```python
from build123d import *

# Parameters (mm, degrees)
SKETCH1_W           = 31.8
SKETCH1_H           = 48
BOSS_EXTRUDE1_DEPTH = 15.8
SKETCH2_R           = 7.62
CUT_EXTRUDE1_DEPTH  = 12.7
SKETCH3_R           = 2.77815
SKETCH3_R_2         = 1.8415
CUT_EXTRUDE2_DEPTH  = 12.7
CUT_EXTRUDE3_DEPTH  = 1.905
SKETCH5_R           = 2.4
BOSS_EXTRUDE2_DEPTH = 1.905
SKETCH6_W           = 29.36
SKETCH6_H           = 13.36
SKETCH6_R           = 3.2605
CUT_EXTRUDE4_DEPTH  = 1.905


with BuildPart() as part:
    # Sketch1 → Boss-Extrude1 (new body)
    with BuildSketch(Plane.XY):
        Rectangle(SKETCH1_W, SKETCH1_H)
    extrude(amount=BOSS_EXTRUDE1_DEPTH)

    # Sketch2 → Cut-Extrude1 (cut)
    with BuildSketch(Plane.XY.offset(15.8)):
        with Locations((0, 8.6)):
            Circle(SKETCH2_R)
        with BuildLine():
            Line((4.7625, -4.1), (4.7625, -16.8))
            ThreePointArc((4.7625, -16.8), (0, -21.5625), (-4.7625, -16.8))
            Line((-4.7625, -16.8), (-4.7625, -4.1))
            ThreePointArc((-4.7625, -4.1), (0, 0.6625), (4.7625, -4.1))
        make_face()
    extrude(amount=-CUT_EXTRUDE1_DEPTH, mode=Mode.SUBTRACT)

    # Sketch3 → Cut-Extrude2 (cut)
    with BuildSketch(Plane(origin=(0, 0, 0), x_dir=(-1, 0, 0), z_dir=(0, 0, -1))):
        with Locations((0, 8.6)):
            Circle(SKETCH3_R)
        with Locations((0, -4.1)):
            Circle(SKETCH3_R_2)
        with Locations((0, -16.8)):
            Circle(SKETCH3_R_2)
    extrude(amount=-CUT_EXTRUDE2_DEPTH, mode=Mode.SUBTRACT)

    # Sketch4 → Cut-Extrude3 (cut)
    with BuildSketch(Plane(origin=(0, 0, 0), x_dir=(-1, 0, 0), z_dir=(0, 0, -1))):
        with BuildLine():
            Line((4.7625, -16.8), (4.7625, -4.1))
            ThreePointArc((4.7625, -4.1), (0, 0.6625), (-4.7625, -4.1))
            Line((-4.7625, -4.1), (-4.7625, -16.8))
            ThreePointArc((-4.7625, -16.8), (0, -21.5625), (4.7625, -16.8))
        make_face()
    extrude(amount=-CUT_EXTRUDE3_DEPTH, mode=Mode.SUBTRACT)

    # Sketch5 → Boss-Extrude2 (add)
    with BuildSketch(Plane.XZ.offset(24)):
        with Locations((-12, 11.9)):
            Circle(SKETCH5_R)
        with Locations((-12, 3.9)):
            Circle(SKETCH5_R)
        with Locations((-4, 11.9)):
            Circle(SKETCH5_R)
        with Locations((-4, 3.9)):
            Circle(SKETCH5_R)
        with Locations((4, 11.9)):
            Circle(SKETCH5_R)
        with Locations((4, 3.9)):
            Circle(SKETCH5_R)
        with Locations((12, 11.9)):
            Circle(SKETCH5_R)
        with Locations((12, 3.9)):
            Circle(SKETCH5_R)
    extrude(amount=BOSS_EXTRUDE2_DEPTH)

    # Sketch6 → Cut-Extrude4 (cut)
    with BuildSketch(Plane(origin=(0, 24, 0), x_dir=(1, 0, 0), z_dir=(0, 1, 0))):
        with Locations((0, -7.9)):
            Rectangle(SKETCH6_W, SKETCH6_H)
        with Locations((-8, -7.9)):
            Circle(SKETCH6_R, mode=Mode.SUBTRACT)
        with Locations((0, -7.9)):
            Circle(SKETCH6_R, mode=Mode.SUBTRACT)
        with Locations((8, -7.9)):
            Circle(SKETCH6_R, mode=Mode.SUBTRACT)
    extrude(amount=-CUT_EXTRUDE4_DEPTH, mode=Mode.SUBTRACT)


solid = part.part
```
Verification items for the finished model (mm, model axes). A direction names the side the tool comes from. Give positions to 0.01 mm unless a question says otherwise; leave off trailing zeros. Order: outer loops, then holes, each group sorted by start corner. A loop starts at its lowest first (then second) coordinate and runs counter-clockwise, first axis right, second up. Notation, with made-up numbers: (30.5, -28.5) - (71.5, -28.5) arc R14 cw to (71.5, -15.5) - close; hole circle Ø10 at (84, -26). An arc over 180 degrees is marked (long way). Answer as CSV lines item,"result". Start each with the question number.
Item 1: Access from +Z, -Z, +X, -X, +Y, -Y to the whole of each face (thin tool, end or side, straight path). Record for faces 1 (the face through (11.48, -24.939, 1.557)), 2 (the face through (-14.68, 23, 8)), 3 (the face through (4.762, -10, 1)).
Item 2: Section check A-A, the plane y = 8.6. Record the boundary of the cut face in (x, z), plus the area to 3 significant figures.
Item 3: Section check B-B, the plane z = 11.9. State how many separate pieces and enclosed holes the cut face has, plus the area to 3 significant figures.
Item 4: Material ranges on L1, parallel to Y at x = 0, z = 7.25; L2, parallel to Y at x = 0, z = 1.45 (1 decimal); L3, parallel to Y at x = 0, z = 2.55 (1 decimal), recorded low to high.
Item 5: Section check C-C, the plane x = -13. Record the boundary of the cut face in (y, z) (3 decimals).
Item 6: Mould release check, pull along Y, two halves, no side actions. Record for faces 4 (the face through (0, -10, 3.1)), 5 (the face through (0, 23, 14.58)), 6 (the face through (0, 24, 8)): released by +Y, released by -Y, zero draft, split by the parting line, or undercut.
Item 7: Gauge pin test, flat ends, axial feed: pin 1 (8 mm diameter, centred on x = -6, z = 12.5, fed in from +Y); pin 2 (7.5 mm diameter, centred on x = -0.5, y = -8.5, fed in from +Z); pin 3 (2 mm diameter, centred on x = -0.5, z = 7, fed in from -Y); pin 4 (3.5 mm diameter, centred on x = 0, y = -4.1, fed in from +Z). Record the tip position at first contact, or that the pin passes through.
Filled in:
1,face 1,"-Y"
1,face 2,"+Y"
1,face 3,"-Z"
2,outline,"(-15.9, 0) - (-2.78, 0) - (-2.78, 3.1) - (-7.62, 3.1) - (-7.62, 15.8) - (-15.9, 15.8) - close; (2.78, 0) - (15.9, 0) - (15.9, 15.8) - (7.62, 15.8) - (7.62, 3.1) - (2.78, 3.1) - close"
2,area,"292 mm^2"
3,separate pieces,"1"
3,enclosed holes,"2"
3,area,"1,130 mm^2"
4,L1,"-24 to -21.56, 0.66 to 0.98, 16.22 to 24"
4,L2,"-24 to -21.6, 0.7 to 5.8, 11.4 to 22.1"
4,L3,"-24 to -18.6, -15 to -5.9, -2.3 to 5.8, 11.4 to 22.1"
5,outline,"(-25.905, 1.718) - (-24, 1.718) - (-24, 0) - (24, 0) - (24, 1.22) - (22.095, 1.22) - (22.095, 14.58) - (24, 14.58) - (24, 15.8) - (-24, 15.8) - (-24, 14.082) - (-25.905, 14.082) - (-25.905, 9.718) - (-24, 9.718) - (-24, 6.082) - (-25.905, 6.082) - close"
6,face 4,"undercut"
6,face 5,"zero draft"
6,face 6,"released by +Y"
7,pin 1,"y = 24"
7,pin 2,"z = 3.1"
7,pin 3,"y = -24"
7,pin 4,"through"
